from build123d import *

# Parameters (mm, degrees)
F0_W     = 6
F0_H     = 10
F0_W_2   = 3
F0_W_3   = 2
F0_W_4   = 8
F1_DEPTH = 3
F2_DEPTH = 43
F3_DEPTH = 44


with BuildPart() as f1:
    # F0 (on Top) → F1 (new body)
    with BuildSketch(Plane.XY):
        with Locations((-12, 0)):
            Rectangle(F0_W, F0_H)
        with Locations((-7.5, 0)):
            Rectangle(F0_W_2, F0_H)
        with Locations((-5, 0)):
            Rectangle(F0_W_3, F0_H)
        Rectangle(F0_W_4, F0_H)
        with Locations((5, 0)):
            Rectangle(F0_W_3, F0_H)
        with Locations((7.5, 0)):
            Rectangle(F0_W_2, F0_H)
        with Locations((12, 0)):
            Rectangle(F0_W, F0_H)
    extrude(amount=F1_DEPTH)

    # F0 (on Top) → F2 (join)
    with BuildSketch(Plane.XY):
        with Locations((7.5, 0)):
            Rectangle(F0_W_2, F0_H)
        with Locations((-7.5, 0)):
            Rectangle(F0_W_2, F0_H)
    extrude(amount=F2_DEPTH)

    # F0 (on Top) → F3 (join)
    with BuildSketch(Plane.XY):
        with Locations((-5, 0)):
            Rectangle(F0_W_3, F0_H)
        with Locations((5, 0)):
            Rectangle(F0_W_3, F0_H)
    extrude(amount=F3_DEPTH)


solid = f1.part
Part model, mm, in its own coordinate system. A direction names the side the tool comes from. Coordinates: 2 decimals unless noted, no trailing zeros. Loops run counter-clockwise (first coordinate to the right, second up) from the corner with the lowest first, then second, coordinate; pieces in that order, holes last. Notation, with made-up numbers: (-19.75, 53.5) -> (25.25, 53.5) arc R27 ccw to (25.25, 84.5) -> close; hole circle Ø7 at (-26.5, -31.75). An arc over 180 degrees is marked (long way). Use a Markdown table: item, result. Add a question column.
Item 1: Band-saw the part on C-C on x = -7.25. Write the cut outline in (y, z).
Item 2: Band-saw the part on D-D on x = 3.5. Write the cut outline in (y, z), plus the area to 3 significant figures.
Item 3: Probe probe 1 along X at (y, z) = (1, 26); probe 2 along Z at (x, y) = (0.5, -0.25); probe 3 along Z at (x, y) = (-7.75, -1). List the from-to ranges inside material, lowest first.
Item 4: Band-saw the part on A-A on z = 9.5. Write the cut outline in (x, y).
Item 5: Flat gauge pins, fed straight in: P1, Ø1.5, axis at y = 4, z = 9, coming from the -X side; P2, Ø2.5, axis at x = -7, y = 2, coming from the +Z side; P3, Ø0.8, axis at y = -1.5, z = 43.5, coming from the +X side; P4, Ø1.5, axis at x = 7.5, y = 0.5, coming from the +Z side. Where does each tip first touch, or does it go through?
Item 6: Which spindle directions (+Z, -Z, +X, -X, +Y, -Y) get a long thin tool onto all of the face, cutting with end or side? Do faces 1 (the flat face through (-15, 0, 1)), 2 (the flat face through (-8, 0, 43)), 3 (the flat face through (5, 0, 44)), 4 (the flat face through (12, 0, 3)), 5 (the flat face through (-4, 0, 23)). Say none if no direction does.
Item 7: Pull direction X, two halves, no side cores. Call faces 6 (the flat face through (4, 0, 23)), 7 (the flat face through (-12, 0, 3)), 8 (the flat face through (6, -0.1, 43.5)): +X half, -X half, draft (parallel to the pull), parting line (faces both ways), or undercut.
Item 8: Band-saw the part on B-B on y = 1.5. Write the cut outline in (x, z).
Geometry says:
| question | item | result |
|---|---|---|
| 1 | outline | (-5, 0) -> (5, 0) -> (5, 43) -> (-5, 43) -> close |
| 2 | outline | (-5, 0) -> (5, 0) -> (5, 3) -> (-5, 3) -> close |
| 2 | area | 30.0 mm² |
| 3 | probe 1 | -9 to -4, 4 to 9 |
| 3 | probe 2 | 0 to 3 |
| 3 | probe 3 | 0 to 43 |
| 4 | outline | (-9, -5) -> (-4, -5) -> (-4, 5) -> (-9, 5) -> close; (4, -5) -> (9, -5) -> (9, 5) -> (4, 5) -> close |
| 5 | P1 | x = -9 |
| 5 | P2 | z = 44 |
| 5 | P3 | x = 6 |
| 5 | P4 | z = 43 |
| 6 | face 1 | +Z, -Z, -X, +Y, -Y |
| 6 | face 2 | +Z, -X, +Y, -Y |
| 6 | face 3 | +Z, +X, -X, +Y, -Y |
| 6 | face 4 | +Z, +X, +Y, -Y |
| 6 | face 5 | +Z, +Y, -Y |
| 7 | face 6 | undercut |
| 7 | face 7 | draft |
| 7 | face 8 | +X half |
| 8 | outline | (-15, 0) -> (15, 0) -> (15, 3) -> (9, 3) -> (9, 43) -> (6, 43) -> (6, 44) -> (4, 44) -> (4, 3) -> (-4, 3) -> (-4, 44) -> (-6, 44) -> (-6, 43) -> (-9, 43) -> (-9, 3) -> (-15, 3) -> close |
